Could you check a few things on this drawing? It's one solid part, dimensions in mm from its lowest x, y, z. A direction names the side the tool comes from. Round coordinates to 2 decimals unless told otherwise and drop trailing zeros. Write each loop counter-clockwise with the first axis right and the second up, starting at its lowest first coordinate (ties: lowest second). Pieces come first, ordered by that corner, then holes. Notation, with made-up numbers: M -32.5,79.5 L 18.5,79.5 A20 ccw 18.5,97.5 Z; hole C 6,-11 d3. An arc over 180 degrees is marked long. One line per item, written item: value. Start each with the question number.
(1) I'm going to push flat-ended pins straight in: pin 1 Ø16 at (y, z) = (8, 20) entering from +X; pin 2 Ø6.5 at (x, z) = (34.5, 17.5) entering from +Y; pin 3 Ø3 at (x, z) = (21, 11.5) entering from -Y; pin 4 Ø4 at (x, y) = (6, 50.5) entering from +Z. Where does each tip first touch, or does it pass through?
(2) Thinking about a two-plate mould opening in X: for the marked faces 1, 2, 3 and 4, which applies, released by +X, released by -X, zero draft, split by the parting line, or undercut?
(3) I want a section at A-A on z = 15. Please give me the cut outline in (x, y), and give its area (3 significant figures).
(4) If I drill on L1, parallel to Y at x = 22, z = 13.25; L2, parallel to X at y = 21, z = 10.5; L3, parallel to Z at x = 34, y = 24, over which ranges is the centre line in solid material (lowest first)?
(5) I want a section at C-C on x = 19.5. Please give me the cut outline in (y, z).
(6) I want a section at B-B on y = 14. Please give me the cut outline in (x, z).
(7) Which directions (+Z, -Z, +X, -X, +Y, -Y) give clear straight access to the entire face, cutting with the end or side of a thin tool? Please do the marked faces 5, 6, 7, 8 and 9.
(8) I want a section at D-D on y = 75.5. Please give me the cut outline in (x, z), and give its area (3 significant figures).
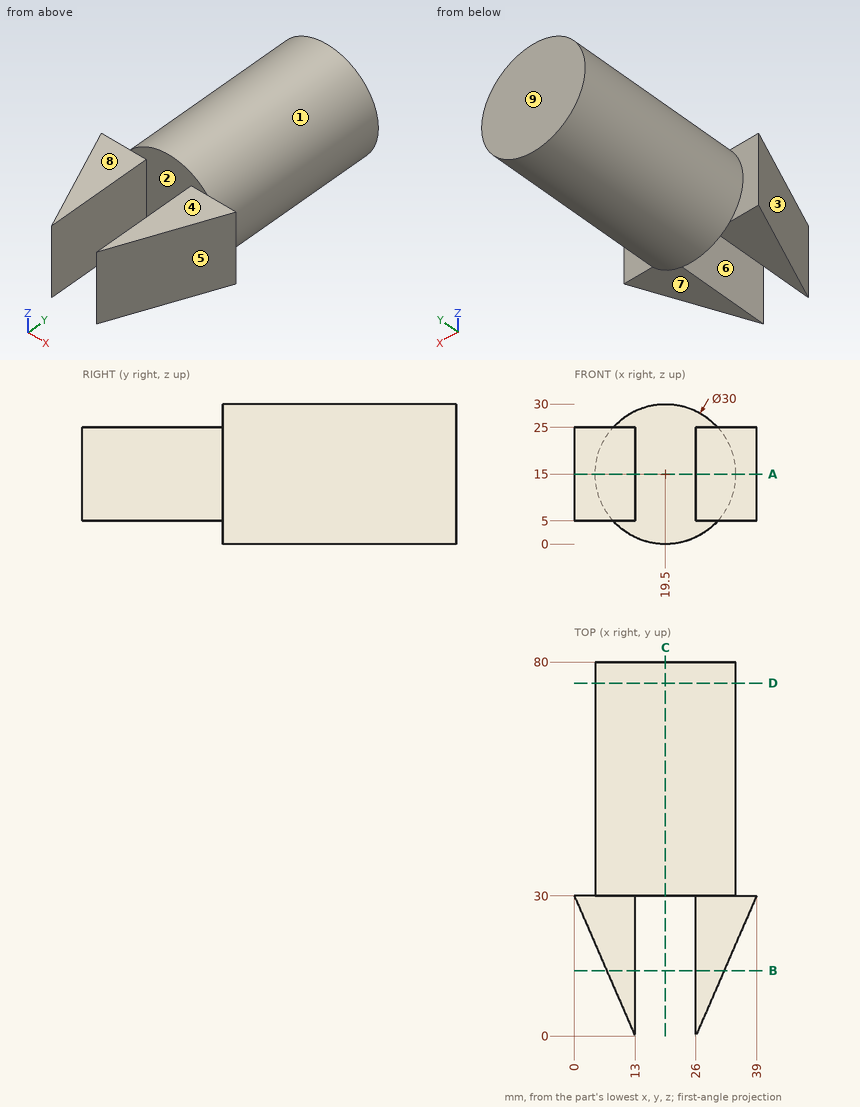
Found:
1. pin 1: stops at x = 32.93
1. pin 2: stops at y = 80
1. pin 3: stops at y = 30
1. pin 4: stops at z = 24.63
2. face 1: split by the parting line
2. face 2: undercut
2. face 3: released by -X
2. face 4: zero draft
3. outline: M 0,30 L 13,0 L 13,30 L 26,30 L 26,0 L 39,30 L 34.5,30 L 34.5,80 L 4.5,80 L 4.5,30 Z
3. area: 1,890 mm²
4. L1: y = 30 to 80
4. L2: x = 3.9 to 13, 26 to 35.1
4. L3: z = 5 to 25
5. outline: M 30,0 L 80,0 L 80,30 L 30,30 Z
6. outline: M 6.93,5 L 13,5 L 13,25 L 6.93,25 Z; M 26,5 L 32.07,5 L 32.07,25 L 26,25 Z
7. face 5: +Z, -Z, +X, -Y
7. face 6: +Z, -Z, -Y
7. face 7: -Z, +X, -X, -Y
7. face 8: +Z, +X, -X, -Y
7. face 9: +Z, -Z, +X, -X, +Y
8. outline: C 19.5,15 d30
8. area: 707 mm²
